The figure shows three views and two pictorial views of one solid part (mm, origin at its lowest corner). Answer the questions. A direction names the side the tool comes from. Give positions to 0.01 mm unless a question says otherwise; leave off trailing zeros. Order: outer loops, then holes, each group sorted by start corner. A loop starts at its lowest first (then second) coordinate and runs counter-clockwise, first axis right, second up. Notation, with made-up numbers: (-11.5, 22.25) - (45.5, 22.25) arc R7 ccw to (45.5, 27.25) - close; hole circle Ø1 at (47.5, 64). An arc over 180 degrees is marked (long way). Answer as a JSON object with one key per item and string values. Group by question number.
Q1. A cutting plane is placed at A-A, the plane z = 1.45. Give the vertices of the cut face in (x, y).
Q2. Consider line 1 (X direction, y = 4, z = 1.9); line 2 (X direction, y = 4, z = 2.6); line 3 (X direction, y = 5.75, z = 2). Determine where each line is inside the solid, lowest interval first.
Q3. A cutting plane is placed at D-D, the plane z = 2.25. Give the vertices of the cut face in (x, y).
Q4. A cutting plane is placed at B-B, the plane y = 4. Give the vertices of the cut face in (x, z).
Q5. For the marked faces 1, 2 and 3, determine the directions among +Z, -Z, +X, -X, +Y, -Y from which every point of the face is accessible in a straight line to the end or side of a thin tool.
Q6. A cutting plane is placed at C-C, the plane x = 12.25. Give the vertices of the cut face in (y, z).
Q7. The mould has two halves that part along X. Classify the marked faces 4, 5 and 6: released by +X, released by -X, zero draft, split by the parting line, or undercut.
Q8. Given pin 1 (2.5 mm diameter, centred on x = 8, y = 4.04, fed in from +Z); pin 2 (1.5 mm diameter, centred on y = 6.5, z = 1, fed in from -X), each flat-ended and moving along its own axis, determine where each tip first touches the part or whether it passes through.
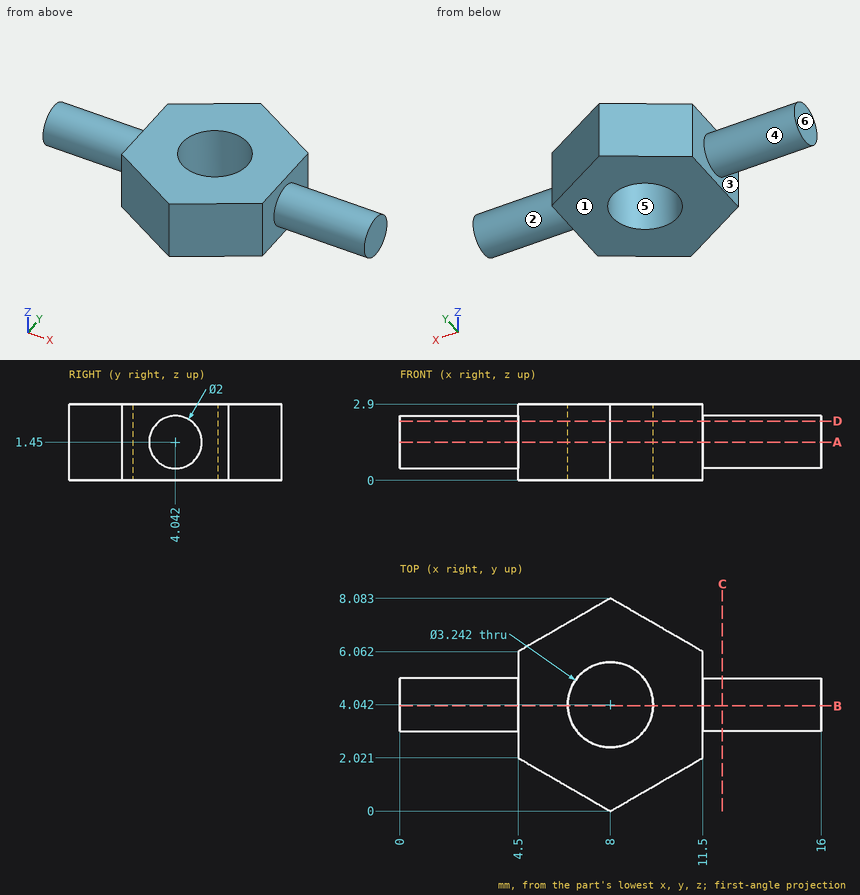
Reply:
{
 "1": {"outline": "(0, 3.04) - (4.5, 3.04) - (4.5, 2.02) - (8, 0) - (11.5, 2.02) - (11.5, 3.04) - (16, 3.04) - (16, 5.04) - (11.5, 5.04) - (11.5, 6.06) - (8, 8.08) - (4.5, 6.06) - (4.5, 5.04) - (0, 5.04) - close; hole circle Ø3.24 at (8, 4.04)"},
 "2": {"line 1": "x = 0 to 6.38, 9.62 to 16", "line 2": "x = 4.5 to 6.38, 9.62 to 11.5", "line 3": "x = 4.5 to 11.5"},
 "3": {"outline": "(0, 3.44) - (4.5, 3.44) - (4.5, 2.02) - (8, 0) - (11.5, 2.02) - (11.5, 3.44) - (16, 3.44) - (16, 4.64) - (11.5, 4.64) - (11.5, 6.06) - (8, 8.08) - (4.5, 6.06) - (4.5, 4.64) - (0, 4.64) - close; hole circle Ø3.24 at (8, 4.04)"},
 "4": {"outline": "(0, 0.45) - (4.5, 0.45) - (4.5, 0) - (6.38, 0) - (6.38, 2.9) - (4.5, 2.9) - (4.5, 2.45) - (0, 2.45) - close; (9.62, 0) - (11.5, 0) - (11.5, 0.45) - (16, 0.45) - (16, 2.45) - (11.5, 2.45) - (11.5, 2.9) - (9.62, 2.9) - close"},
 "5": {"face 1": "-Z, +X, -X, +Y, -Y", "face 2": "+X", "face 3": "-X"},
 "6": {"outline": "circle Ø2 at (4.04, 1.45)"},
 "7": {"face 4": "zero draft", "face 5": "undercut", "face 6": "released by -X"},
 "8": {"pin 1": "passes through", "pin 2": "stops at x = 4.5"}
}
